CAD build for the part. Positions are in the model's coordinates, mm. Face numbers are marked on the shaded views. A direction names the side the tool comes from. Give positions to 0.01 mm unless a question says otherwise; leave off trailing zeros. Loops run counter-clockwise (first coordinate to the right, second up) from the corner with the lowest first, then second, coordinate; pieces in that order, holes last.
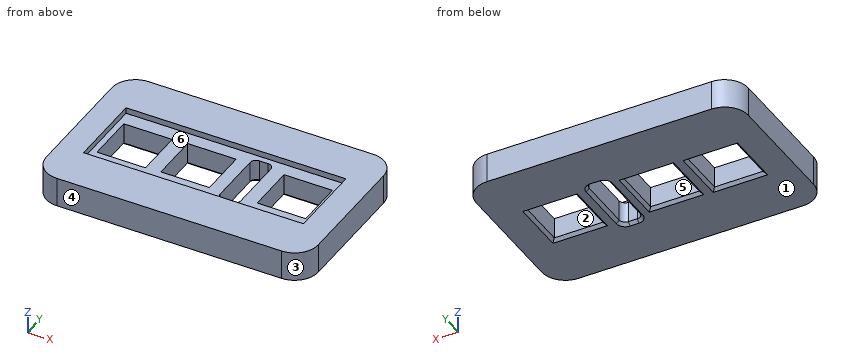
```python
from build123d import *

# Parameters (mm, degrees)
F0_W     = 58.42
F0_H     = 35.56
F1_DEPTH = 6.35
F4_W     = 10.414
F4_H     = 10.414
F4_W_2   = 4.445
F4_H_2   = 14.224
F5_DEPTH = 25.4
F6_R     = 1.27
F3_W     = 47.244
F3_H     = 16.51
F7_DEPTH = 1.27
F8_R     = 5.08
F9_SIZE  = 0.635


with BuildPart() as f1:
    # F0 (on Top) → F1 (new body)
    with BuildSketch(Plane.XY):
        with Locations((-70.023337, -16.211975)):
            Rectangle(F0_W, F0_H)
    extrude(amount=F1_DEPTH)

    # F4 (on face) → F5 (cut)
    with BuildSketch(Plane.XY.offset(6.35)):
        with Locations((-87.295337, -16.211975)):
            Rectangle(F4_W, F4_H)
        with Locations((-73.706337, -15.957975)):
            Rectangle(F4_W, F4_H)
        with Locations((-53.005337, -15.957975)):
            Rectangle(F4_W, F4_H)
        with Locations((-63.482837, -16.211975)):
            Rectangle(F4_W_2, F4_H_2)
    extrude(amount=-F5_DEPTH, mode=Mode.SUBTRACT)

    # F6
    f6_edges = [f1.edges().sort_by_distance(p)[0] for p in [
        (-65.705337, -9.099975, 3.175),
        (-61.260337, -9.099975, 3.175),
        (-61.260337, -23.323975, 3.175),
        (-65.705337, -23.323975, 3.175),
    ]]
    fillet(f6_edges, radius=F6_R)

    # F3 (on face) → F7 (cut)
    with BuildSketch(Plane.XY.offset(6.35)):
        with Locations((-70.150337, -16.084975)):
            Rectangle(F3_W, F3_H)
    extrude(amount=-F7_DEPTH, mode=Mode.SUBTRACT)

    # F8
    f8_edges = [f1.edges().sort_by_distance(p)[0] for p in [
        (-40.813337, -33.991975, 3.175),
        (-40.813337, 1.568025, 3.175),
        (-99.233337, -33.991975, 3.175),
        (-99.233337, 1.568025, 3.175),
    ]]
    fillet(f8_edges, radius=F8_R)

    # F9
    f9_edges = [f1.edges().sort_by_distance(p)[0] for p in [
        (-87.295337, -21.418975, 0),
        (-87.295337, -11.004975, 0),
        (-82.088337, -16.211975, 0),
        (-92.502337, -16.211975, 0),
        (-73.706337, -21.164975, 0),
        (-78.913337, -15.957975, 0),
        (-73.706337, -10.750975, 0),
        (-68.499337, -15.957975, 0),
        (-65.705337, -16.211975, 0),
        (-58.212337, -15.957975, 0),
        (-53.005337, -21.164975, 0),
        (-47.798337, -15.957975, 0),
        (-53.005337, -10.750975, 0),
    ]]
    chamfer(f9_edges, length=F9_SIZE)


solid = f1.part
```
1. Saw through at C-C, the plane z = 1.5. List the corners of the cut face in (x, y).
Responses:
outline: (-99.23, -28.91) arc R5.08 ccw to (-94.15, -33.99) - (-45.89, -33.99) arc R5.08 ccw to (-40.81, -28.91) - (-40.81, -3.51) arc R5.08 ccw to (-45.89, 1.57) - (-94.15, 1.57) arc R5.08 ccw to (-99.23, -3.51) - close; hole (-92.5, -21.42) - (-82.09, -21.42) - (-82.09, -11) - (-92.5, -11) - close; hole (-78.91, -21.16) - (-68.5, -21.16) - (-68.5, -10.75) - (-78.91, -10.75) - close; hole (-65.71, -22.05) arc R1.27 ccw to (-64.44, -23.32) - (-62.53, -23.32) arc R1.27 ccw to (-61.26, -22.05) - (-61.26, -10.37) arc R1.27 ccw to (-62.53, -9.1) - (-64.44, -9.1) arc R1.27 ccw to (-65.71, -10.37) - close; hole (-58.21, -21.16) - (-47.8, -21.16) - (-47.8, -10.75) - (-58.21, -10.75) - close
2. Drop flat-ended pins along their axis: pin 1 (12 mm diameter, centred on x = -62.5, y = -22, fed in from -Z); pin 2 (5 mm diameter, centred on x = -57.5, y = -18.5, fed in from +Z). Give the stop position or say it passes through.
Responses:
pin 1: stops at z = 0
pin 2: stops at z = 5.08
3. Tool access for the marked faces 4, 5 and 6: list every direction of +Z, -Z, +X, -X, +Y, -Y with a clear straight run to the whole face (end or side of a thin tool).
Responses:
face 4: +Z, -Z, +X, -X, -Y
face 5: +Z, -Z
face 6: +Z
4. Pull direction Y, two halves, no side cores. Call the marked faces 1, 2 and 3: released by +Y, released by -Y, zero draft, split by the parting line, or undercut.
Responses:
face 1: zero draft
face 2: undercut
face 3: released by -Y
5. Probe line 1 along X through (y, z) = (-12, 2); line 2 along Y through (x, z) = (-50.5, 4.25); line 3 along Y through (x, z) = (-84, 5). List the from-to ranges inside material, lowest first.
Responses:
line 1: x = -99.23 to -92.5, -82.09 to -78.91, -68.5 to -65.71, -61.26 to -58.21, -47.8 to -40.81
line 2: y = -33.99 to -21.16, -10.75 to 1.57
line 3: y = -33.99 to -21.42, -11 to 1.57
6. Saw through at D-D, the plane x = -80.5. List the corners of the cut face in (y, z), and give its area (3 significant figures).
Responses:
outline: (-33.99, 0) - (1.57, 0) - (1.57, 6.35) - (-7.83, 6.35) - (-7.83, 5.08) - (-24.34, 5.08) - (-24.34, 6.35) - (-33.99, 6.35) - close
area: 205 mm2
7. Saw through at A-A, the plane x = -48.5. List the corners of the cut face in (y, z) (3 decimals), and give its area (3 significant figures).
Responses:
outline: (-33.992, 0) - (-21.8, 0) - (-21.165, 0.635) - (-21.165, 5.08) - (-24.34, 5.08) - (-24.34, 6.35) - (-33.992, 6.35) - close; (-10.751, 0.635) - (-10.116, 0) - (1.568, 0) - (1.568, 6.35) - (-7.83, 6.35) - (-7.83, 5.08) - (-10.751, 5.08) - close
area: 152 mm2
8. Saw through at B-B, the plane y = -19. Count the separate pieces of the cut face and the enclosed holes in it, and give its area (3 significant figures).
Responses:
separate pieces: 5
enclosed holes: 0
area: 128 mm2
